The model under review builds one solid part; all positions refer to its coordinate system, in mm. A direction names the side the tool comes from. Give positions to 0.01 mm unless a question says otherwise; leave off trailing zeros. Order: outer loops, then holes, each group sorted by start corner. A loop starts at its lowest first (then second) coordinate and runs counter-clockwise, first axis right, second up. Notation, with made-up numbers: (78, 23.5) -> (87, 23.5) arc R33 cw to (87, 57.5) -> close; hole circle Ø8 at (70, 3). An arc over 180 degrees is marked (long way). Use one line per item in the form item = value.
Autodesk Inventor part; units mm, degrees
ref_plane "YZ Plane" through (0, 0, 0) normal (1, 0, 0) x (0, 1, 0)
ref_plane "XZ Plane" through (0, 0, 0) normal (0, 1, 0) x (-1, 0, 0)
ref_plane "XY Plane" through (0, 0, 0) normal (0, 0, 1) x (1, 0, 0)
sketch "Sketch1" plane through (0, 0, 0) normal (0, 0, 1) x (1, 0, 0)
  line L0 (0, 0) -> (12.7, 0)
  line L1 (12.7, 0) -> (12.7, 1.27)
  line L2 (12.7, 1.27) -> (1.27, 1.27)
  line L3 (1.27, 1.27) -> (1.27, 12.7)
  line L4 (1.27, 12.7) -> (0, 12.7)
  line L5 (0, 12.7) -> (0, 0)
  dimension "d0" = 12.7
  dimension "d1" = 1.27
extrude "Extrusion1" add sketch "Sketch1" along normal blind 482.6
fillet "Fillet1" radius 1.27 4 edges at (12.7, 1.27, 241.3) (1.27, 1.27, 241.3) (1.27, 12.7, 241.3) (0, 0, 241.3)
sketch "Sketch2" plane through (2.54, 1.27, 482.6) normal (0, 1, 0) x (1, 0, 0)
  line L0 (0, 0) -> (0, 482.6)
  line L1 (8.89, 482.6) -> (8.89, 0)
  line L2 (8.89, 482.6) -> (0, 482.6)
  circle A0 centre (3.81, 476.25) radius 2.4892
  line L3 (-2.54, 482.6) -> (-2.54, 0)
  line L4 (8.89, 241.3) -> (0, 241.3) construction
  circle A1 centre (3.81, 6.35) radius 2.4892
  dimension "d6" = 4.9784
  dimension "d7" = 6.35
  dimension "d8" = 6.35
extrude "Extrusion2" cut sketch "Sketch2" against normal blind 25.4
equation "\"d8\" = d7"
properties part number ".05 in Aluminum Angle (19 in)"
1. Add section C-C on y = 7.5. Give the boundary of the cut face in (x, z).
Values:
outline = (0, 0) -> (1.27, 0) -> (1.27, 482.6) -> (0, 482.6) -> close
2. Tool access review of faces 1 (the face through (1, 4, 482.6)), 2 (the face through (7, 1.27, 238)): name each direction out of +Z, -Z, +X, -X, +Y, -Y from which nothing blocks a thin tool from reaching the whole face with its end or side.
Values:
face_1 = +Z, +X, -X, +Y, -Y
face_2 = +Z, -Z, +X, +Y
3. For pin 1 Ø7 at (y, z) = (8.5, 144) entering from +X; pin 2 Ø4.5 at (x, z) = (6, 247) entering from +Y, all flat-tipped, find the tip position at first contact; note any pin that passes through.
Values:
pin_1 = 1.27
pin_2 = 1.27
4. Add section A-A on x = 6.35. Give the boundary of the cut face in (y, z).
Values:
outline = (0, 0) -> (1.27, 0) -> (1.27, 3.86) -> (0, 3.86) -> close; (0, 8.84) -> (1.27, 8.84) -> (1.27, 473.76) -> (0, 473.76) -> close; (0, 478.74) -> (1.27, 478.74) -> (1.27, 482.6) -> (0, 482.6) -> close
5. For L1, parallel to Z at x = 6.35, y = 1; L2, parallel to X at y = 5.25, z = 412.5; L3, parallel to X at y = 1, z = 476.25, list the stretches that pass through material, from the lowest coordinate up.
Values:
L1 = 0 to 3.86, 8.84 to 473.76, 478.74 to 482.6
L2 = 0 to 1.27
L3 = 0.03 to 3.86, 8.84 to 12.21
